Verification items for this drawing (mm, ordinates from the low corner). A direction names the side the tool comes from. Coordinates: 2 decimals unless noted, no trailing zeros. Order: outer loops, then holes, each group sorted by start corner. A loop starts at its lowest first (then second) coordinate and runs counter-clockwise, first axis right, second up.
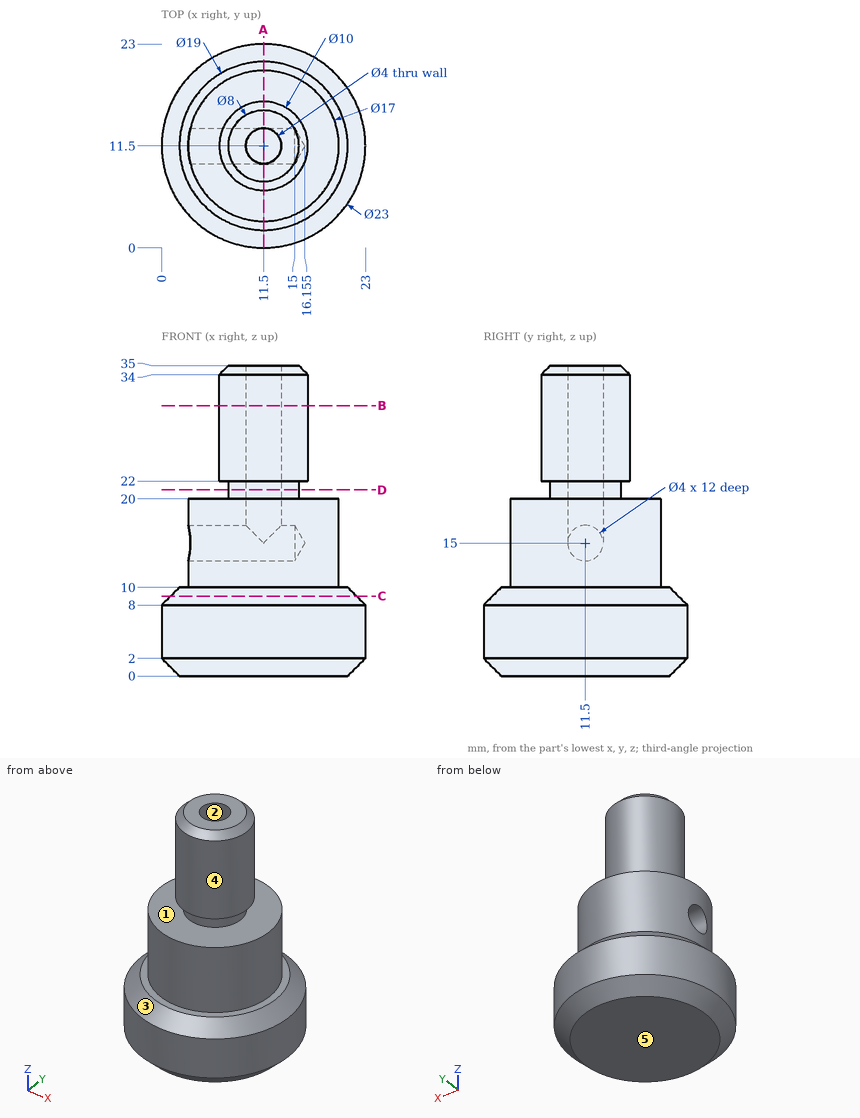
(1) Cross-section at C-C (z = 9). Enter the section's corners in (x, y), and give its area (3 significant figures).
Filled in:
outline: circle Ø21 at (11.5, 11.5)
area: 346 mm2
(2) Cross-section at D-D (z = 21). Enter the section's corners in (x, y).
Filled in:
outline: circle Ø8 at (11.5, 11.5); hole circle Ø4 at (11.5, 11.5)
(3) Thickness scan on probe 1 along Z at (x, y) = (8.5, 11.5); probe 2 along X at (y, z) = (11.5, 29.5); probe 3 along Y at (x, z) = (11.75, 15). Record the ranges inside material, lowest first.
Filled in:
probe 1: z = 0 to 13, 17 to 35
probe 2: x = 6.5 to 9.5, 13.5 to 16.5
probe 3: y = 3 to 9.5, 13.5 to 20
(4) Release check for a two-part mould opening along X. For the marked faces 1, 2 and 3 record: +X half, -X half, draft (parallel to the pull), parting line (faces both ways), or undercut.
Filled in:
face 1: draft
face 2: undercut
face 3: parting line
(5) Tool access check on the marked faces 4 and 5. Record the directions out of +Z, -Z, +X, -X, +Y, -Y that give a thin tool (end or side, any length) a straight path to the whole face; none if there is none.
Filled in:
face 4: +Z
face 5: -Z, +X, -X, +Y, -Y
(6) Cross-section at A-A (x = 11.5). Enter the section's corners in (y, z), and give its area (3 significant figures).
Filled in:
outline: (0, 2) - (2, 0) - (21, 0) - (23, 2) - (23, 8) - (21, 10) - (20, 10) - (20, 20) - (15.5, 20) - (15.5, 22) - (16.5, 22) - (16.5, 34) - (15.5, 35) - (13.5, 35) - (13.5, 15) arc R2 cw to (9.5, 15) - (9.5, 35) - (7.5, 35) - (6.5, 34) - (6.5, 22) - (7.5, 22) - (7.5, 20) - (3, 20) - (3, 10) - (2, 10) - (0, 8) - close
area: 451 mm2
(7) Cross-section at B-B (z = 30.5). Enter the section's corners in (x, y).
Filled in:
outline: circle Ø10 at (11.5, 11.5); hole circle Ø4 at (11.5, 11.5)
(8) Go/stop test with flat-tipped pins: P1, Ø3, axis at y = 11.5, z = 15, coming from the +X side; P2, Ø4, axis at x = 12, z = 23.5, coming from the +Y side; P3, Ø4, axis at x = 19.5, z = 9.5, coming from the -Y side. Record where each tip stops, or that it passes through.
Filled in:
P1: stops at x = 20
P2: stops at y = 16.5
P3: stops at y = 2.14
